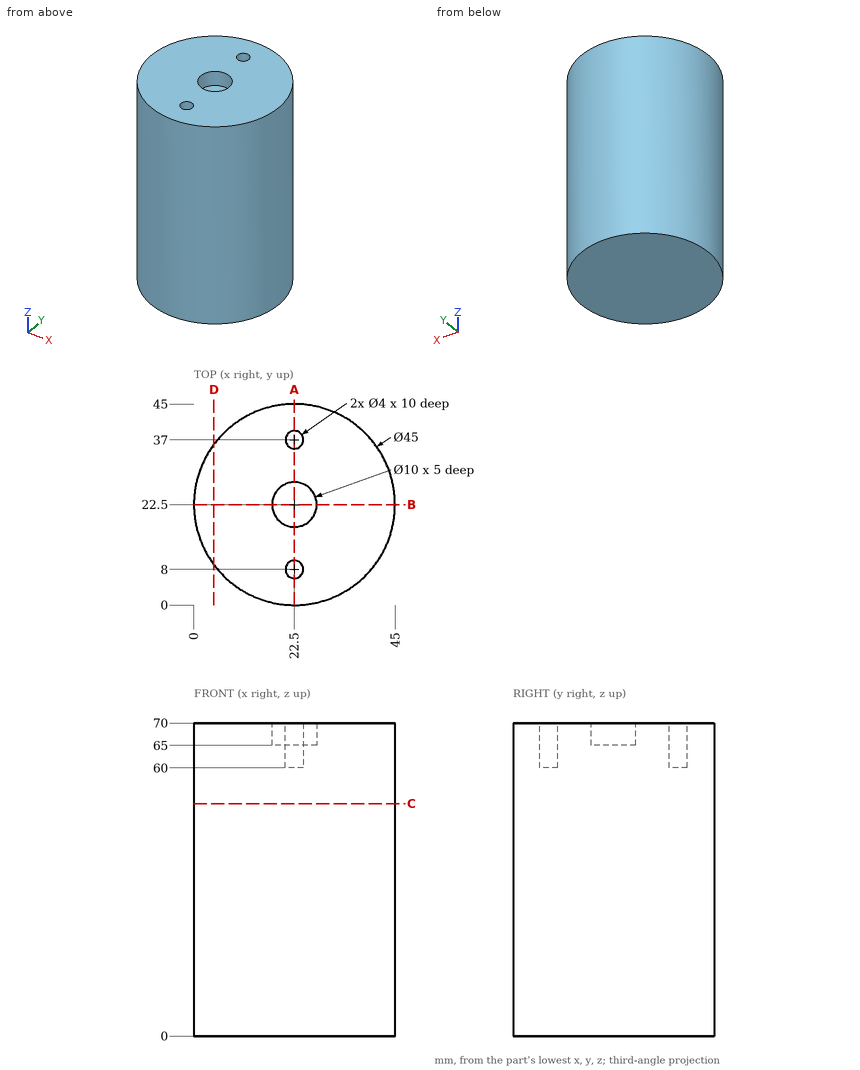
Job drawing, mm, ordinate dimensions from the low corner. One solid piece. Coordinates: 2 decimals unless noted, no trailing zeros. Order: outer loops, then holes, each group sorted by start corner. A loop starts at its lowest first (then second) coordinate and runs counter-clockwise, first axis right, second up. Notation, with made-up numbers: (37, 70) - (92, 70) arc R28 cw to (92, 104) - close; hole circle Ø11 at (29.25, 79). An arc over 180 degrees is marked (long way). Write each question's results on one line, items separated by ' | '. Start each with the question number.
Item 1: Band-saw the part on D-D on x = 4.5. Write the cut outline in (y, z), and give its area (3 significant figures).
Item 2: Band-saw the part on B-B on y = 22.5. Write the cut outline in (x, z).
Item 3: Wall check: probe 1 along Y at (x, z) = (22.5, 64); probe 2 along Y at (x, z) = (22, 66); probe 3 along Y at (x, z) = (22, 62). Give the ranges that are in metal, low to high. Write a range as [from, to].
Item 4: Band-saw the part on C-C on z = 52. Write the cut outline in (x, y).
Item 5: Band-saw the part on A-A on x = 22.5. Write the cut outline in (y, z).
Item 6: Flat gauge pins, fed straight in: pin 1 (3 mm diameter, centred on y = 5.5, z = 18.5, fed in from -X); pin 2 (10 mm diameter, centred on x = 22, z = 23, fed in from +Y); pin 3 (1 mm diameter, centred on y = 30.5, z = 62, fed in from -X). Where does each tip first touch, or does it go through?
Numbers:
1) outline: (9, 0) - (36, 0) - (36, 70) - (9, 70) - close | area: 1,890 mm^2
2) outline: (0, 0) - (45, 0) - (45, 70) - (27.5, 70) - (27.5, 65) - (17.5, 65) - (17.5, 70) - (0, 70) - close
3) probe 1: [0, 6], [10, 35], [39, 45] | probe 2: [0.01, 6.06], [9.94, 17.53], [27.47, 35.06], [38.94, 44.99] | probe 3: [0.01, 6.06], [9.94, 35.06], [38.94, 44.99]
4) outline: circle Ø45 at (22.5, 22.5)
5) outline: (0, 0) - (45, 0) - (45, 70) - (39, 70) - (39, 60) - (35, 60) - (35, 70) - (27.5, 70) - (27.5, 65) - (17.5, 65) - (17.5, 70) - (10, 70) - (10, 60) - (6, 60) - (6, 70) - (0, 70) - close
6) pin 1: x = 6.19 | pin 2: y = 45 | pin 3: x = 1.29
